from build123d import *

# Parameters (mm, degrees)
SKETCH_1_W          = 5
SKETCH_1_H          = 410
EXTRUDE_1_DEPTH     = 53
CUT_EXTRUDE_1_REACH = 401.01
CUT_EXTRUDE_2_REACH = 401.01
CUT_EXTRUDE_3_REACH = 401.01
SKETCH_4_R          = 4


with BuildPart() as part:
    # 草图1 → 凸台-拉伸1 (new body)
    with BuildSketch(Plane(origin=(0, 0, 0), x_dir=(1, 0, 0), z_dir=(0, 1, 0))):
        with Locations((-0.791139241, 190.443037975)):
            Rectangle(SKETCH_1_W, SKETCH_1_H)
    extrude(amount=EXTRUDE_1_DEPTH)

    # 草图2 → 切除-拉伸1 (cut, up to next)
    with BuildSketch(Plane(origin=(1.708860759, 0, 0), x_dir=(0, 0, -1), z_dir=(1, 0, 0)), mode=Mode.PRIVATE) as cut_extrude_1_sk1:
        with BuildLine():
            Line((58.443037975, 44.280521885), (28.443037975, 44.280521885))
            ThreePointArc((28.443037975, 44.280521885), (25.47355986, 47.25), (28.443037975, 50.219478115))
            Line((28.443037975, 50.219478115), (58.443037975, 50.219478115))
            ThreePointArc((58.443037975, 50.219478115), (61.41251609, 47.25), (58.443037975, 44.280521885))
        make_face()
    cut_extrude_1_tool1 = extrude(cut_extrude_1_sk1.sketch, amount=-CUT_EXTRUDE_1_REACH, mode=Mode.PRIVATE) & part.part
    # 草图2 → 切除-拉伸1 (cut, up to next)
    with BuildSketch(Plane(origin=(1.708860759, 0, 0), x_dir=(0, 0, -1), z_dir=(1, 0, 0)), mode=Mode.PRIVATE) as cut_extrude_1_sk2:
        with BuildLine():
            Line((58.443037975, 3.2), (28.443037975, 3.2))
            ThreePointArc((28.443037975, 3.2), (25.893037975, 5.75), (28.443037975, 8.3))
            Line((28.443037975, 8.3), (58.443037975, 8.3))
            ThreePointArc((58.443037975, 8.3), (60.993037975, 5.75), (58.443037975, 3.2))
        make_face()
    cut_extrude_1_tool2 = extrude(cut_extrude_1_sk2.sketch, amount=-CUT_EXTRUDE_1_REACH, mode=Mode.PRIVATE) & part.part
    # 草图2 → 切除-拉伸1 (cut, up to next)
    with BuildSketch(Plane(origin=(1.708860759, 0, 0), x_dir=(0, 0, -1), z_dir=(1, 0, 0)), mode=Mode.PRIVATE) as cut_extrude_1_sk3:
        with BuildLine():
            Line((348.443037975, 49.8), (388.443037975, 49.8))
            ThreePointArc((388.443037975, 49.8), (390.993037975, 47.25), (388.443037975, 44.7))
            Line((388.443037975, 44.7), (348.443037975, 44.7))
            ThreePointArc((348.443037975, 44.7), (345.893037975, 47.25), (348.443037975, 49.8))
        make_face()
    cut_extrude_1_tool3 = extrude(cut_extrude_1_sk3.sketch, amount=-CUT_EXTRUDE_1_REACH, mode=Mode.PRIVATE) & part.part
    # 草图2 → 切除-拉伸1 (cut, up to next)
    with BuildSketch(Plane(origin=(1.708860759, 0, 0), x_dir=(0, 0, -1), z_dir=(1, 0, 0)), mode=Mode.PRIVATE) as cut_extrude_1_sk4:
        with BuildLine():
            Line((348.443037975, 8.3), (388.443037975, 8.3))
            ThreePointArc((388.443037975, 8.3), (390.993037975, 5.75), (388.443037975, 3.2))
            Line((388.443037975, 3.2), (348.443037975, 3.2))
            ThreePointArc((348.443037975, 3.2), (345.893037975, 5.75), (348.443037975, 8.3))
        make_face()
    cut_extrude_1_tool4 = extrude(cut_extrude_1_sk4.sketch, amount=-CUT_EXTRUDE_1_REACH, mode=Mode.PRIVATE) & part.part
    add(cut_extrude_1_tool1.solids().sort_by_distance((1.708861, 47.25, -43.443038))[0], mode=Mode.SUBTRACT)
    add(cut_extrude_1_tool2.solids().sort_by_distance((1.708861, 5.75, -43.443038))[0], mode=Mode.SUBTRACT)
    add(cut_extrude_1_tool3.solids().sort_by_distance((1.708861, 47.25, -368.443038))[0], mode=Mode.SUBTRACT)
    add(cut_extrude_1_tool4.solids().sort_by_distance((1.708861, 5.75, -368.443038))[0], mode=Mode.SUBTRACT)

    # 草图3 → 切除-拉伸2 (cut, up to next)
    with BuildSketch(Plane(origin=(1.708860759, 0, 0), x_dir=(0, 0, -1), z_dir=(1, 0, 0)), mode=Mode.PRIVATE) as cut_extrude_2_sk1:
        Polygon((22.443037975, 26.5), (22.443037975, 38.5), (377.443037975, 38.5), (377.443037975, 14.5), (22.443037975, 14.5), align=None)
    cut_extrude_2_tool1 = extrude(cut_extrude_2_sk1.sketch, amount=-CUT_EXTRUDE_2_REACH, mode=Mode.PRIVATE) & part.part
    add(cut_extrude_2_tool1.solids().sort_by_distance((1.708861, 26.5, -199.943038))[0], mode=Mode.SUBTRACT)

    # 草图4 → 切除-拉伸3 (cut, up to next)
    with BuildSketch(Plane(origin=(1.708860759, 0, 0), x_dir=(0, 0, -1), z_dir=(1, 0, 0)), mode=Mode.PRIVATE) as cut_extrude_3_sk1:
        with Locations((-4.556962025, 41.5)):
            Circle(SKETCH_4_R)
    cut_extrude_3_tool1 = extrude(cut_extrude_3_sk1.sketch, amount=-CUT_EXTRUDE_3_REACH, mode=Mode.PRIVATE) & part.part
    # 草图4 → 切除-拉伸3 (cut, up to next)
    with BuildSketch(Plane(origin=(1.708860759, 0, 0), x_dir=(0, 0, -1), z_dir=(1, 0, 0)), mode=Mode.PRIVATE) as cut_extrude_3_sk2:
        with Locations((15.443037975, 41.5)):
            Circle(SKETCH_4_R)
    cut_extrude_3_tool2 = extrude(cut_extrude_3_sk2.sketch, amount=-CUT_EXTRUDE_3_REACH, mode=Mode.PRIVATE) & part.part
    # 草图4 → 切除-拉伸3 (cut, up to next)
    with BuildSketch(Plane(origin=(1.708860759, 0, 0), x_dir=(0, 0, -1), z_dir=(1, 0, 0)), mode=Mode.PRIVATE) as cut_extrude_3_sk3:
        with Locations((15.443037975, 11.5)):
            Circle(SKETCH_4_R)
    cut_extrude_3_tool3 = extrude(cut_extrude_3_sk3.sketch, amount=-CUT_EXTRUDE_3_REACH, mode=Mode.PRIVATE) & part.part
    # 草图4 → 切除-拉伸3 (cut, up to next)
    with BuildSketch(Plane(origin=(1.708860759, 0, 0), x_dir=(0, 0, -1), z_dir=(1, 0, 0)), mode=Mode.PRIVATE) as cut_extrude_3_sk4:
        with Locations((-4.556962025, 11.5)):
            Circle(SKETCH_4_R)
    cut_extrude_3_tool4 = extrude(cut_extrude_3_sk4.sketch, amount=-CUT_EXTRUDE_3_REACH, mode=Mode.PRIVATE) & part.part
    add(cut_extrude_3_tool1.solids().sort_by_distance((1.708861, 41.5, 4.556962))[0], mode=Mode.SUBTRACT)
    add(cut_extrude_3_tool2.solids().sort_by_distance((1.708861, 41.5, -15.443038))[0], mode=Mode.SUBTRACT)
    add(cut_extrude_3_tool3.solids().sort_by_distance((1.708861, 11.5, -15.443038))[0], mode=Mode.SUBTRACT)
    add(cut_extrude_3_tool4.solids().sort_by_distance((1.708861, 11.5, 4.556962))[0], mode=Mode.SUBTRACT)


solid = part.part
The model under review builds one solid part; all positions refer to its coordinate system, in mm. Round coordinates to 2 decimals unless told otherwise and drop trailing zeros. Loops run counter-clockwise (first coordinate to the right, second up) from the corner with the lowest first, then second, coordinate; pieces in that order, holes last. Notation, with made-up numbers: (51, 64) -> (75, 64) arc R17 ccw to (75, 75) -> close; hole circle Ø2 at (-31, -31). An arc over 180 degrees is marked (long way). Write item = value, one per line. Start each with the question number.
Item 1: Take a section at A-A on z = -171. Give the boundary of the cut face in (x, y), plus the area to 3 significant figures.
Item 2: Take a section at B-B on x = -0.2. Count the separate pieces of the cut face and the enclosed holes in it, plus the area to 3 significant figures.
Item 3: Insertion check: pin 1 (5 mm diameter, centred on y = 41.5, z = -15.44, fed in from +X). The pin has a flat end and moves straight along its axis. Give the tip position at first contact, or say it passes through.
Item 4: Take a section at C-C on y = 31.5. Give the boundary of the cut face in (x, z), plus the area to 3 significant figures.
Item 5: Mouldability with a two-part tool opening along Y and no side actions: class faces 1 (the flat face through (1.709, 14, -188)), 2 (the cylindrical face through (-0.76, 14.2, 7.51)) as released by +Y, released by -Y, zero draft, split by the parting line, or undercut.
Item 6: To check wall thickness, follow L1, parallel to Y at x = -0.45, z = -354; L2, parallel to Z at x = 1.25, y = 41; L3, parallel to Z at x = 0.1, y = 36. State the ranges of each line that lie inside material, in increasing order.
Result:
q1.outline = (-3.29, 0) -> (1.71, 0) -> (1.71, 14.5) -> (-3.29, 14.5) -> close; (-3.29, 38.5) -> (1.71, 38.5) -> (1.71, 53) -> (-3.29, 53) -> close
q1.area = 145 mm²
q2.separate_pieces = 1
q2.enclosed_holes = 9
q2.area = 12,200 mm²
q3.pin_1 = through
q4.outline = (-3.29, -395.44) -> (1.71, -395.44) -> (1.71, -377.44) -> (-3.29, -377.44) -> close; (-3.29, -22.44) -> (1.71, -22.44) -> (1.71, 14.56) -> (-3.29, 14.56) -> close
q4.area = 275 mm²
q5.face_1 = zero draft
q5.face_2 = undercut
q6.L1 = 0 to 3.2, 8.3 to 14.5, 38.5 to 44.7, 49.8 to 53
q6.L2 = -395.44 to -19.41, -11.47 to 0.59, 8.53 to 14.56
q6.L3 = -395.44 to -377.44, -22.44 to 14.56
